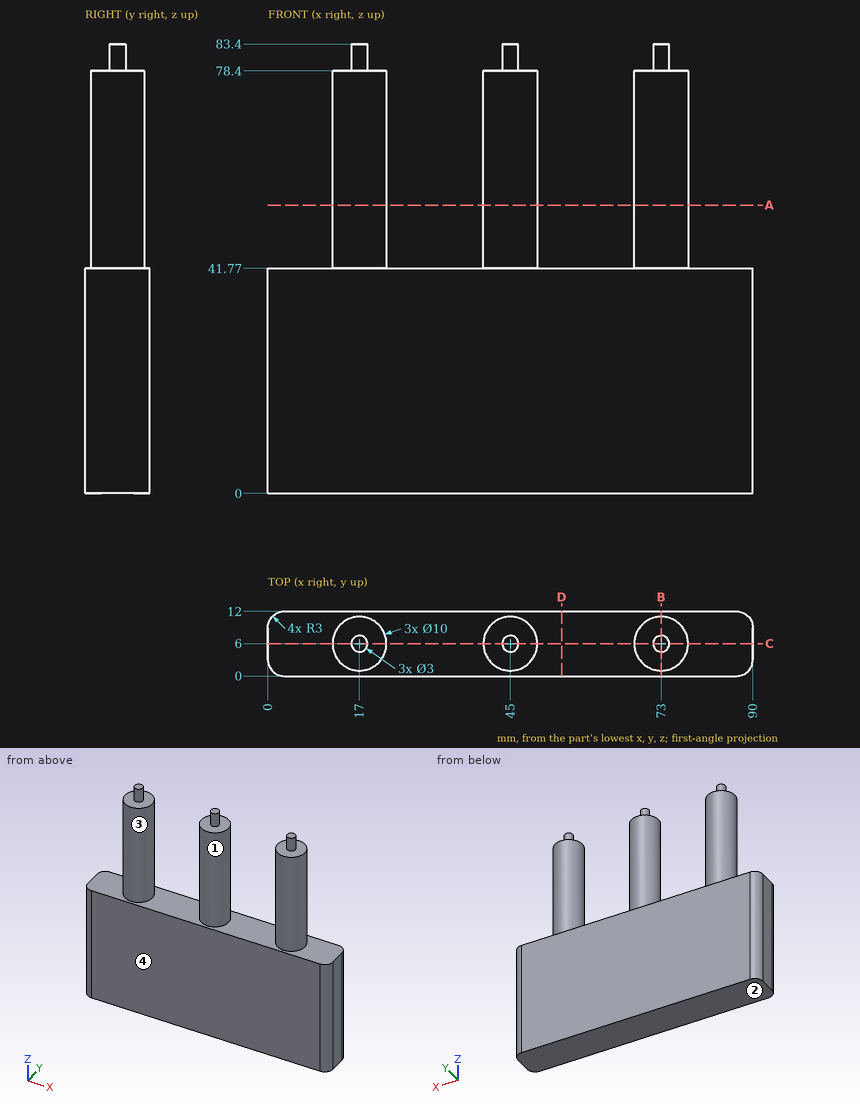
Could you check a few things on this drawing? It's one solid part, dimensions in mm from its lowest x, y, z. A direction names the side the tool comes from. Coordinates: 2 decimals unless noted, no trailing zeros. Loops run counter-clockwise (first coordinate to the right, second up) from the corner with the lowest first, then second, coordinate; pieces in that order, holes last.
1. For P1, Ø1, axis at x = 78, z = 72.5, coming from the -Y side; P2, Ø2, axis at x = 44.5, z = 59.5, coming from the -Y side, each with a flat end and sliding along its axis, tell me the tip position at first contact or that it passes through.
2. Imagine slicing it at C-C (y = 6). Please give me the cut outline in (x, z), and give its area (3 significant figures).
3. Imagine slicing it at A-A (z = 53.5). Please give me the cut outline in (x, y).
4. We'd pull the mould along X, two halves only. Please class the marked faces 3 and 4: released by +X, released by -X, zero draft, split by the parting line, or undercut.
5. I need wall thicknesses on L1, parallel to X at y = 6.25, z = 54.5; L2, parallel to X at y = 3, z = 54; L3, parallel to Z at x = 71, y = 8.25. Which ranges of each line are inside material? Lowest first, please.
6. Imagine slicing it at D-D (x = 54.5). Please give me the cut outline in (y, z).
7. For the marked faces 1 and 2, which set-ups out of +Z, -Z, +X, -X, +Y, -Y let a thin tool reach every point of the face, with its end or its side?
8. Imagine slicing it at B-B (x = 73). Please give me the cut outline in (y, z), and give its area (3 significant figures).
Computed values:
1. P1: stops at y = 3.82
1. P2: stops at y = 1
2. outline: (0, 0) - (90, 0) - (90, 41.77) - (78, 41.77) - (78, 78.4) - (74.5, 78.4) - (74.5, 83.4) - (71.5, 83.4) - (71.5, 78.4) - (68, 78.4) - (68, 41.77) - (50, 41.77) - (50, 78.4) - (46.5, 78.4) - (46.5, 83.4) - (43.5, 83.4) - (43.5, 78.4) - (40, 78.4) - (40, 41.77) - (22, 41.77) - (22, 78.4) - (18.5, 78.4) - (18.5, 83.4) - (15.5, 83.4) - (15.5, 78.4) - (12, 78.4) - (12, 41.77) - (0, 41.77) - close
2. area: 4,900 mm2
3. outline: circle Ø10 at (17, 6); circle Ø10 at (45, 6); circle Ø10 at (73, 6)
4. face 3: undercut
4. face 4: zero draft
5. L1: x = 12.01 to 21.99, 40.01 to 49.99, 68.01 to 77.99
5. L2: x = 13 to 21, 41 to 49, 69 to 77
5. L3: z = 0 to 78.4
6. outline: (0, 0) - (12, 0) - (12, 41.77) - (0, 41.77) - close
7. face 1: +Z
7. face 2: -Z, +X, -X, +Y, -Y
8. outline: (0, 0) - (12, 0) - (12, 41.77) - (11, 41.77) - (11, 78.4) - (7.5, 78.4) - (7.5, 83.4) - (4.5, 83.4) - (4.5, 78.4) - (1, 78.4) - (1, 41.77) - (0, 41.77) - close
8. area: 883 mm2
